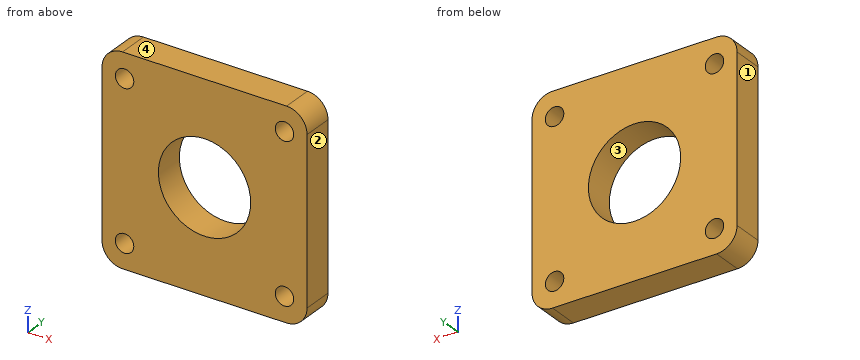
```python
from build123d import *

# Parameters (mm, degrees)
F0_R     = 4.5
F0_R_2   = 22.5
F1_DEPTH = 15


with BuildPart() as f1:
    # F0 (on Front) → F1 (new body)
    with BuildSketch(Plane.XZ):
        with BuildLine():
            Line((40, 50), (-40, 50))
            ThreePointArc((-40, 50), (-47.071068, 47.071068), (-50, 40))
            Line((-50, 40), (-50, -40))
            ThreePointArc((-50, -40), (-47.071068, -47.071068), (-40, -50))
            Line((-40, -50), (40, -50))
            ThreePointArc((40, -50), (47.071068, -47.071068), (50, -40))
            Line((50, -40), (50, 40))
            ThreePointArc((50, 40), (47.071068, 47.071068), (40, 50))
        make_face()
        with Locations((-39, -38)):
            Circle(F0_R, mode=Mode.SUBTRACT)
        with Locations((39, -38)):
            Circle(F0_R, mode=Mode.SUBTRACT)
        with Locations((-39, 38)):
            Circle(F0_R, mode=Mode.SUBTRACT)
        Circle(F0_R_2, mode=Mode.SUBTRACT)
        with Locations((39, 38)):
            Circle(F0_R, mode=Mode.SUBTRACT)
    extrude(amount=F1_DEPTH)


solid = f1.part
```
Here's how the part is built. I have some questions about the finished solid (model axes, mm). Face numbers are marked on the shaded views. Give positions to 0.01 mm unless a question says otherwise; leave off trailing zeros. Write each loop counter-clockwise with the first axis right and the second up, starting at its lowest first coordinate (ties: lowest second). Pieces come first, ordered by that corner, then holes. Notation, with made-up numbers: (77, -25) -> (84, -25) arc R14 cw to (84, -14) -> close; hole circle Ø8 at (33, -34.75). An arc over 180 degrees is marked (long way). Use one line per item in the form item = value.
1) Suppose I cut it at A-A (z = -38). Please give me the cut outline in (x, y).
Verdict:
outline = (-50, -15) -> (-43.5, -15) -> (-43.5, 0) -> (-50, 0) -> close; (-34.5, -15) -> (34.5, -15) -> (34.5, 0) -> (-34.5, 0) -> close; (43.5, -15) -> (50, -15) -> (50, 0) -> (43.5, 0) -> close
2) Suppose I cut it at D-D (z = 0). Please give me the cut outline in (x, y).
Verdict:
outline = (-50, -15) -> (-22.5, -15) -> (-22.5, 0) -> (-50, 0) -> close; (22.5, -15) -> (50, -15) -> (50, 0) -> (22.5, 0) -> close
3) I'm going to push a flat-ended pin straight in: pin 1 (5 mm diameter, centred on x = -12, z = 18.5, fed in from +Y). Where does the tip first touch, or does it pass through?
Verdict:
pin_1 = 0
4) Suppose I cut it at B-B (y = -6.25). Please give me the cut outline in (x, z).
Verdict:
outline = (-50, -40) arc R10 ccw to (-40, -50) -> (40, -50) arc R10 ccw to (50, -40) -> (50, 40) arc R10 ccw to (40, 50) -> (-40, 50) arc R10 ccw to (-50, 40) -> close; hole circle Ø9 at (-39, -38); hole circle Ø9 at (-39, 38); hole circle Ø45 at (0, 0); hole circle Ø9 at (39, -38); hole circle Ø9 at (39, 38)
5) If I drill on L1, parallel to Z at x = 39, y = -3; L2, parallel to X at y = -4.5, z = 36; L3, parallel to Z at x = 35, y = -14, over which ranges is the centre line in solid material (lowest first)? Write a range as [from, to].
Verdict:
L1 = [-50, -42.5], [-33.5, 33.5], [42.5, 50]
L2 = [-50, -43.03], [-34.97, 34.97], [43.03, 50]
L3 = [-50, -40.06], [-35.94, 35.94], [40.06, 50]
6) We'd pull the mould along X, two halves only. Please class the marked faces 1, 2, 3 and 4: +X half, -X half, draft (parallel to the pull), parting line (faces both ways), or undercut.
Verdict:
face_1 = -X half
face_2 = +X half
face_3 = undercut
face_4 = draft
7) Suppose I cut it at C-C (x = 1.5). Please give me the cut outline in (y, z).
Verdict:
outline = (-15, -50) -> (0, -50) -> (0, -22.45) -> (-15, -22.45) -> close; (-15, 22.45) -> (0, 22.45) -> (0, 50) -> (-15, 50) -> close
